Geometry check sheet. Reference: the model listing, model coordinates, mm. A direction names the side the tool comes from. Coordinates: 2 decimals unless noted, no trailing zeros. Loops run counter-clockwise (first coordinate to the right, second up) from the corner with the lowest first, then second, coordinate; pieces in that order, holes last. Notation, with made-up numbers: (-23.5, 82.5) - (16.5, 82.5) arc R15 cw to (16.5, 109.5) - close; hole circle Ø2 at (-22, -38). An arc over 180 degrees is marked (long way). One line per item, written item: value.
from build123d import *

# Parameters (mm, degrees)
BOSS_EXTRUDE1_DEPTH                 = 6.35
F_9_64_0_14063_DIAMETER_HOLE1_D     = 3.572002
F_9_64_0_14063_DIAMETER_HOLE1_DEPTH = 12.7
F_9_64_0_14063_DIAMETER_HOLE1_TIP   = 1.073137666


with BuildPart() as part:
    # Sketch1 → Boss-Extrude1 (new body)
    with BuildSketch(Plane.XY):
        Polygon((-39.37, 8.89), (-39.37, 0), (-57.15, 0), (-57.15, 38.1), (57.15, 38.1), (57.15, 0), (39.37, 0), (39.37, 8.89), (25.4, 8.89), (25.4, 0), (-25.4, 0), (-25.4, 8.89), align=None)
    extrude(amount=BOSS_EXTRUDE1_DEPTH)

    # 9/64 (0.14063) Diameter Hole1
    with Locations(Plane.XZ.offset(-8.89)):
        with Locations((-32.766, 3.175), (32.766, 3.175)):
            Hole(F_9_64_0_14063_DIAMETER_HOLE1_D / 2, depth=F_9_64_0_14063_DIAMETER_HOLE1_DEPTH)
            with Locations((0, 0, -(F_9_64_0_14063_DIAMETER_HOLE1_DEPTH + F_9_64_0_14063_DIAMETER_HOLE1_TIP / 2))):  # 118° drill point
                Cone(0, F_9_64_0_14063_DIAMETER_HOLE1_D / 2, F_9_64_0_14063_DIAMETER_HOLE1_TIP, mode=Mode.SUBTRACT)


solid = part.part
(1) Cross-section at C-C on x = -36.5. Record the cut outline in (y, z), and give its area (3 significant figures).
Reply:
outline: (8.89, 0) - (38.1, 0) - (38.1, 6.35) - (8.89, 6.35) - close
area: 185 mm2
(2) Cross-section at B-B on y = 12. Record the cut outline in (x, z) (3 decimals).
Reply:
outline: (-57.15, 0) - (57.15, 0) - (57.15, 6.35) - (-57.15, 6.35) - close; hole circle Ø3.572 at (-32.766, 3.175); hole circle Ø3.572 at (32.766, 3.175)
(3) Material ranges on probe 1 along X at (y, z) = (13, 2.25); probe 2 along Y at (x, z) = (39, 2); probe 3 along Y at (x, z) = (34, 2), recorded low to high. Write a range as from..to.
Reply:
probe 1: -57.15..-34.29, -31.24..31.24, 34.29..57.15
probe 2: 8.89..38.1
probe 3: 21.64..38.1
(4) Go/stop test with flat-tipped pins: pin 1 Ø1.9 at (x, z) = (31, 3.5) entering from -Y; pin 2 Ø3 at (x, z) = (32.766, 3.175) entering from -Y. Record where each tip stops, or that it passes through.
Reply:
pin 1: y = 8.89
pin 2: y = 21.76
(5) Release check for a two-part mould opening along Z. For faces 1 (the face through (-34.416, 15.329, 2.491)), 2 (the face through (1, 19, 6.35)), 3 (the face through (0, 0, 3)) record: pulls with the +Z half, pulls with the -Z half, needs draft (parallel to the pull), parting line crosses it, or undercut.
Reply:
face 1: undercut
face 2: pulls with the +Z half
face 3: needs draft
(6) Cross-section at A-A on y = 7.5. Record the cut outline in (x, z).
Reply:
outline: (-57.15, 0) - (-39.37, 0) - (-39.37, 6.35) - (-57.15, 6.35) - close; (-25.4, 0) - (25.4, 0) - (25.4, 6.35) - (-25.4, 6.35) - close; (39.37, 0) - (57.15, 0) - (57.15, 6.35) - (39.37, 6.35) - close
(7) Access from +Z, -Z, +X, -X, +Y, -Y to the whole of each face (thin tool, end or side, straight path). Record for faces 4 (the face through (34.55, 15.33, 3.25)), 5 (the face through (-39.37, 5, 3)), 6 (the face through (57.15, 19, 3)).
Reply:
face 4: -Y
face 5: +Z, -Z, -Y
face 6: +Z, -Z, +X, +Y, -Y
